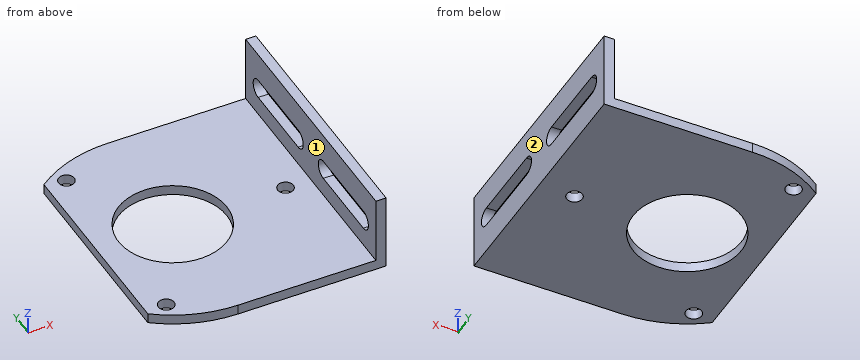
Autodesk Inventor part; units mm, degrees
ref_plane "YZ Plane" through (0, 0, 0) normal (1, 0, 0) x (0, 1, 0)
ref_plane "XZ Plane" through (0, 0, 0) normal (0, 1, 0) x (-1, 0, 0)
ref_plane "XY Plane" through (0, 0, 0) normal (0, 0, 1) x (1, 0, 0)
sketch "Sketch2" plane through (0, 0, 0) normal (0, 1, 0) x (-1, 0, 0)
  line L0 (38.1, 25.4) -> (-38.1, 25.4)
  line L1 (-38.1, 25.4) -> (-38.1, -25.4)
  line L2 (-38.1, -25.4) -> (38.1, -25.4)
  line L3 (38.1, -25.4) -> (38.1, 25.4)
  line L4 (34.798, 22.098) -> (-34.798, 22.098)
  line L5 (-34.798, 22.098) -> (-34.798, -22.098)
  line L6 (-34.798, -22.098) -> (34.798, -22.098)
  line L7 (34.798, -22.098) -> (34.798, 22.098)
  line L8 (0, -35.56) -> (0, 35.56)
  line L9 (-53.34, 0) -> (53.34, 0)
  point P0 (0, 0)
  dimension "d0" = 3.302
  dimension "d1" = 76.2
  dimension "d2" = 50.8
extrude "Extrusion1" add sketch "Sketch2" along normal mid plane 82.55 contours L3 L9 L7 L4 L8 L0 | L8 L4 L5 L9 L1 L0 | L3 L2 L8 L6 L7 L9 | L9 L5 L6 L8 L2 L1
sketch "Sketch4" plane through (-34.798, -41.275, -22.098) normal (0, 0, 1) x (1, 0, 0)
  line L0 (0, 0) -> (0, 82.55)
  line L1 (69.596, 0) -> (0, 0)
  line L2 (69.596, 0) -> (69.596, 82.55)
  line L3 (0, 82.55) -> (69.596, 82.55)
  arc A0 (0, 8.3506) -> (0, 74.1994) centre (24.892, 41.275) ccw
  line L4 (-18.542, 41.275) -> (88.138, 41.275)
  line L5 (0, 8.3506) -> (0, 74.1994)
  line L6 (72.898, 82.55) -> (-3.302, 82.55) construction
  circle A1 centre (24.892, 41.275) radius 17.526
  line L7 (-3.302, 0) -> (72.898, 0)
  line L8 (24.892, 0) -> (-3.302, 0)
  line L9 (-3.302, 0) -> (-3.302, 82.55)
  line L10 (-3.302, 0) -> (-3.302, 82.55)
  line L11 (-3.302, 82.55) -> (24.892, 82.55)
  circle A2 centre (61.4172, 41.275) radius 2.54
  circle A3 centre (6.6294, 72.9068) radius 2.54
  circle A4 centre (6.6294, 9.6432) radius 2.54
  point P0 (34.798, 41.275)
  dimension "d9" = 44.704
  dimension "d13" = 35.052
  dimension "d26" = 36.5252
  dimension "d27" = 5.08
  dimension "d30" = 360
extrude "Extrusion3" cut sketch "Sketch4" along normal up to surface (47.498 mm away) contours L7 L9 L4 L0 | L0 A0 L1 | L4 L9 L11 L0 | L0 L3 A0 | A1 L4 | L4 A1 | A2 L4 | L4 A2 | A3 | A4
extrude "Extrusion4" cut sketch "Sketch4" against normal up to surface (3.302 mm away) contours L7 L9 L4 L0 | L0 A0 L1 | L4 L9 L11 L0 | L0 L3 A0 | A1 L4 | L4 A1 | A2 L4 | L4 A2 | A3 | A4
sketch "Sketch5" plane through (38.1, -41.275, -25.4) normal (1, 0, 0) x (0, 0, -1)
  line L0 (0, 0) -> (0, 82.55)
  line L1 (-50.8, 82.55) -> (0, 82.55)
  line L2 (-50.8, 0) -> (-50.8, 82.55)
  line L3 (0, 0) -> (-50.8, 0)
  line L4 (-25.4, 0) -> (-25.4, 82.55)
  line L5 (-50.8, 82.55) -> (0, 82.55)
  point P0 (-25.4, 41.275)
  dimension "d18" = 25.4
extrude "Extrusion5" cut sketch "Sketch5" against normal up to surface (72.898 mm away) contours L3 L2 L1 L4
sketch "Sketch6" plane through (34.798, -41.275, -22.098) normal (-1, 0, 0) x (0, 0, 1)
  line L0 (22.098, 0) -> (22.098, 82.55)
  line L1 (0, 0) -> (0, 82.55)
  line L2 (44.196, 0) -> (0, 0)
  arc A0 (12.573, 74.6125) -> (6.223, 74.6125) centre (9.398, 74.6125) ccw
  arc A1 (6.223, 7.9375) -> (12.573, 7.9375) centre (9.398, 7.9375) ccw
  arc A2 (6.223, 49.2125) -> (12.573, 49.2125) centre (9.398, 49.2125) ccw
  arc A3 (12.573, 33.3375) -> (6.223, 33.3375) centre (9.398, 33.3375) ccw
  line L3 (12.573, 33.3375) -> (12.573, 7.9375)
  line L4 (6.223, 7.9375) -> (6.223, 33.3375)
  line L5 (12.573, 49.2125) -> (12.573, 74.6125)
  line L6 (6.223, 74.6125) -> (6.223, 49.2125)
  line L7 (22.098, 41.275) -> (0, 41.275) construction
  line L8 (6.223, 61.9125) -> (12.573, 61.9125) construction
  line L9 (0, 82.55) -> (22.098, 82.55) construction
  line L10 (0, 82.55) -> (44.196, 82.55) construction
  line L11 (9.398, 74.6125) -> (9.398, 49.2125) construction
  point P0 (22.098, 41.275)
  dimension "d21" = 6.35
  dimension "d22" = 25.4
  dimension "d23" = 12.7
extrude "Extrusion6" cut sketch "Sketch6" against normal up to next
equation "\"d0\" = WallThickness"
equation "\"d3\" = DiameterMotor"
equation "\"d13\" = InnerHole"
equation "\"d26\" = Distance2Screw"
equation "\"WallThickness\" = 3.302"
equation "\"DiameterMotor\" = 82.55"
equation "\"InnerHole\" = 35.052"
equation "\"Distance2Screw\" = 36.5252"
equation "\"ScrewDiameter\" = 5.08"
properties part number "CIM Bracket"
The listing builds one solid part. Answer for the finished solid, in the listing's coordinates (mm). Face numbers are marked on the shaded views. A direction names the side the tool comes from. Give positions to 0.01 mm unless a question says otherwise; leave off trailing zeros. Loops run counter-clockwise (first coordinate to the right, second up) from the corner with the lowest first, then second, coordinate; pieces in that order, holes last. Notation, with made-up numbers: (1, 27.25) - (22, 27.25) arc R18 ccw to (22, 37.25) - close; hole circle Ø4 at (-30.75, 6). An arc over 180 degrees is marked (long way). Return JSON: item names as keys, results as strings. Group by question number.
1. Find section D-D (y = 0). Write down the section's boundary in (x, z), then the cut area to 3 significant figures.
2. Given pin 1 Ø4 at (y, z) = (22, -4) entering from -X; pin 2 Ø1 at (x, y) = (23.5, -6) entering from +Z; pin 3 Ø4.5 at (x, y) = (26.62, 0) entering from +Z, each flat-ended and moving along its own axis, determine where each tip first touches the part or whether it passes through.
3. Straight lines are drawn through the part: line 1 (X direction, y = 0, z = -24.2); line 2 (Z direction, x = 35.5, y = -12.5) (3 decimals); line 3 (Z direction, x = -7.5, y = 28). For each, find the intervals that lie inside material, in ascending order. Write a range as [from, to].
4. Find section C-C (x = -9). Write down the section's boundary in (y, z) (3 decimals).
5. Find section A-A (z = -12.7). Write down the section's boundary in (x, y) (1 decimal), then the cut area to 3 significant figures.
6. Which of the six approach directions +Z, -Z, +X, -X, +Y, -Y give full straight-line access (tool end or side, diameter ignored) to the marked faces 1 and 2?
7. Find section B-B (y = -20). Write down the section's boundary in (x, z) (3 decimals).
Verdict:
{
 "1": {"outline": "(-34.8, -25.4) - (-27.43, -25.4) - (-27.43, -22.1) - (-34.8, -22.1) - close; (7.62, -25.4) - (24.08, -25.4) - (24.08, -22.1) - (7.62, -22.1) - close; (29.16, -25.4) - (38.1, -25.4) - (38.1, 0) - (34.8, 0) - (34.8, -22.1) - (29.16, -22.1) - close", "area": "181 mm^2"},
 "2": {"pin 1": "stops at x = 34.8", "pin 2": "stops at z = -22.1", "pin 3": "passes through"},
 "3": {"line 1": "x = [-34.8, -27.43], [7.62, 24.08], [29.16, 38.1]", "line 2": "z = [-25.4, -15.875], [-9.525, 0]", "line 3": "z = [-25.4, -22.1]"},
 "4": {"outline": "(-41.275, -25.4) - (-17.503, -25.4) - (-17.503, -22.098) - (-41.275, -22.098) - close; (17.503, -25.4) - (41.275, -25.4) - (41.275, -22.098) - (17.503, -22.098) - close"},
 "5": {"outline": "(34.8, -41.3) - (38.1, -41.3) - (38.1, -36.5) - (34.8, -36.5) - close; (34.8, -4.8) - (38.1, -4.8) - (38.1, 4.8) - (34.8, 4.8) - close; (34.8, 36.5) - (38.1, 36.5) - (38.1, 41.3) - (34.8, 41.3) - close", "area": "62.9 mm^2"},
 "6": {"face 1": "+Z, -X, +Y, -Y", "face 2": "+Z, -Z, +X, +Y, -Y"},
 "7": {"outline": "(-34.798, -25.4) - (38.1, -25.4) - (38.1, -15.875) - (34.798, -15.875) - (34.798, -22.098) - (-34.798, -22.098) - close; (34.798, -9.525) - (38.1, -9.525) - (38.1, 0) - (34.798, 0) - close"}
}
